from build123d import *

# Parameters (mm, degrees)
SKETCH4_W            = 31.4
SKETCH4_H            = 31.4
SKETCH4_W_2          = 25.4
SKETCH4_H_2          = 25.4
BOSS_EXTRUDE3_DEPTH  = 30
SKETCH5_W            = 31.4
SKETCH5_H            = 31.4
BOSS_EXTRUDE4_DEPTH  = 5
SKETCH6_W            = 31.4
SKETCH6_H            = 8
BOSS_EXTRUDE5_DEPTH  = 5
BOSS_EXTRUDE6_DEPTH  = 8
SKETCH8_R            = 9.5
BOSS_EXTRUDE7_DEPTH  = 8
SKETCH9_W            = 31.4
SKETCH9_H            = 10
BOSS_EXTRUDE8_DEPTH  = 5
SKETCH10_W           = 31.4
SKETCH10_H           = 10
BOSS_EXTRUDE9_DEPTH  = 13
SKETCH11_W           = 6.2
SKETCH11_H           = 10
BOSS_EXTRUDE10_DEPTH = 40
BOSS_EXTRUDE11_DEPTH = 3
SKETCH13_W           = 31.4
SKETCH13_H           = 31.4
CUT_EXTRUDE1_DEPTH   = 31.4
SKETCH15_W           = 31.4
SKETCH15_H           = 13
BOSS_EXTRUDE12_DEPTH = 12
SKETCH17_W           = 8
SKETCH17_H           = 31.4
BOSS_EXTRUDE13_DEPTH = 10
SKETCH18_R           = 3.5
BOSS_EXTRUDE14_DEPTH = 8
SKETCH19_W           = 3.6
SKETCH19_H           = 5
CUT_EXTRUDE2_DEPTH   = 31.4
CUT_EXTRUDE3_START   = 8
SKETCH8_2_R          = 9.5
CUT_EXTRUDE3_DEPTH   = 24
SKETCH20_W           = 8
SKETCH20_H           = 1
CUT_EXTRUDE4_DEPTH   = 26.4


with BuildPart() as part:
    # Sketch4 → Boss-Extrude3 (new body)
    with BuildSketch(Plane.XY):
        Rectangle(SKETCH4_W, SKETCH4_H)
        Rectangle(SKETCH4_W_2, SKETCH4_H_2, mode=Mode.SUBTRACT)
    extrude(amount=BOSS_EXTRUDE3_DEPTH)

    # Sketch5 → Boss-Extrude4 (add)
    with BuildSketch(Plane.XY.offset(30)):
        Rectangle(SKETCH5_W, SKETCH5_H)
    extrude(amount=BOSS_EXTRUDE4_DEPTH)

    # Sketch6 → Boss-Extrude5 (add)
    with BuildSketch(Plane.XY.offset(35)):
        Rectangle(SKETCH6_W, SKETCH6_H)
    extrude(amount=BOSS_EXTRUDE5_DEPTH)

    # Sketch7 → Boss-Extrude6 (add)
    with BuildSketch(Plane.XZ.offset(4)):
        with BuildLine():
            Line((-15.7, 40), (-15.7, 52))
            ThreePointArc((-15.7, 52), (-11.306601718, 62.606601718), (-0.7, 67))
            Line((-0.7, 67), (0.7, 67))
            ThreePointArc((0.7, 67), (11.306601718, 62.606601718), (15.7, 52))
            Line((15.7, 52), (15.7, 40))
            Line((15.7, 40), (-15.7, 40))
        make_face()
    extrude(amount=-BOSS_EXTRUDE6_DEPTH)

    # Sketch8 → Boss-Extrude7 (add)
    with BuildSketch(Plane.XZ.offset(4)):
        with Locations(Location((0, 52, 0), (0, 0, 180))):
            Circle(SKETCH8_R)
    boss_extrude7 = extrude(amount=BOSS_EXTRUDE7_DEPTH)

    # Mirror1: Boss-Extrude7 across plane
    add(boss_extrude7.mirror(Plane.ZX))

    # Sketch9 → Boss-Extrude8 (add)
    with BuildSketch(Plane(origin=(0, 15.7, 0), x_dir=(1, 0, 0), z_dir=(0, 1, 0))):
        with Locations((0, -27)):
            Rectangle(SKETCH9_W, SKETCH9_H)
    extrude(amount=BOSS_EXTRUDE8_DEPTH)

    # Sketch10 → Boss-Extrude9 (add)
    with BuildSketch(Plane(origin=(0, 15.7, 0), x_dir=(1, 0, 0), z_dir=(0, 1, 0))):
        with Locations((0, -17)):
            Rectangle(SKETCH10_W, SKETCH10_H)
    extrude(amount=BOSS_EXTRUDE9_DEPTH)

    # Sketch11 → Boss-Extrude10 (add)
    with BuildSketch(Plane(origin=(0, 20.7, 0), x_dir=(1, 0, 0), z_dir=(0, 1, 0))):
        with Locations((-12.6, -27)):
            Rectangle(SKETCH11_W, SKETCH11_H)
        with Locations((12.6, -27)):
            Rectangle(SKETCH11_W, SKETCH11_H)
    extrude(amount=BOSS_EXTRUDE10_DEPTH)

    # Sketch12 → Boss-Extrude11 (add)
    with BuildSketch(Plane.XY.offset(32)):
        Polygon((-15.7, 60.7), (-9.5, 60.7), (-9.5, 20.7), (9.5, 20.7), (9.5, 60.7), (15.7, 60.7), (15.7, 15.7), (-15.7, 15.7), align=None)
    extrude(amount=BOSS_EXTRUDE11_DEPTH)

    # Sketch13 → Cut-Extrude1 (cut)
    with BuildSketch(Plane.ZY.offset(15.7)):
        with Locations((15.7, 0)):
            Rectangle(SKETCH13_W, SKETCH13_H)
    extrude(amount=-CUT_EXTRUDE1_DEPTH, mode=Mode.SUBTRACT)

    # Sketch15 → Boss-Extrude12 (add)
    with BuildSketch(Plane(origin=(0, 0, 12), x_dir=(-1, 0, 0), z_dir=(0, 0, -1))):
        with Locations((0, 22.2)):
            Rectangle(SKETCH15_W, SKETCH15_H)
    extrude(amount=BOSS_EXTRUDE12_DEPTH)

    # Sketch17 → Boss-Extrude13 (add)
    with BuildSketch(Plane.XZ.offset(-15.7)):
        with Locations((-8, 15.7)):
            Rectangle(SKETCH17_W, SKETCH17_H)
    boss_extrude13 = extrude(amount=BOSS_EXTRUDE13_DEPTH)

    # Sketch18 → Boss-Extrude14 (add)
    with BuildSketch(Plane.ZY.offset(12)):
        with BuildLine():
            Line((31.4, 5.7), (0, 5.7))
            Line((0, 5.7), (0, -13.3))
            ThreePointArc((0, -13.3), (4.393398282, -23.906601718), (15, -28.3))
            Line((15, -28.3), (16.4, -28.3))
            ThreePointArc((16.4, -28.3), (27.006601718, -23.906601718), (31.4, -13.3))
            Line((31.4, -13.3), (31.4, 5.7))
        make_face()
        with Locations((15.7, -13.3)):
            Circle(SKETCH18_R, mode=Mode.SUBTRACT)
    boss_extrude14 = extrude(amount=-BOSS_EXTRUDE14_DEPTH)

    # Mirror3: Boss-Extrude13, Boss-Extrude14 across plane
    add(boss_extrude13.mirror(Plane(origin=(0, 0, 0), x_dir=(0, 0, 1), z_dir=(1, 0, 0))))
    add(boss_extrude14.mirror(Plane(origin=(0, 0, 0), x_dir=(0, 0, 1), z_dir=(1, 0, 0))))

    # Sketch19 → Cut-Extrude2 (cut)
    with BuildSketch(Plane(origin=(15.7, 0, 0), x_dir=(0, 0, -1), z_dir=(1, 0, 0))):
        with Locations((-33.2, -13.2)):
            Rectangle(SKETCH19_W, SKETCH19_H)
    extrude(amount=-CUT_EXTRUDE2_DEPTH, mode=Mode.SUBTRACT)

    # Sketch8_2 → Cut-Extrude3 (cut)
    with BuildSketch(Plane.XZ.offset(4).offset(CUT_EXTRUDE3_START)):
        with Locations(Location((0, 52, 0), (0, 0, 270))):
            Circle(SKETCH8_2_R)
    extrude(amount=-CUT_EXTRUDE3_DEPTH, mode=Mode.SUBTRACT)

    # Sketch20 → Cut-Extrude4 (cut)
    with BuildSketch(Plane.XZ.offset(10.7)):
        with Locations((0, 31.9)):
            Rectangle(SKETCH20_W, SKETCH20_H)
    extrude(amount=-CUT_EXTRUDE4_DEPTH, mode=Mode.SUBTRACT)


solid = part.part
Model file for the job. Use its own axes, mm. A direction names the side the tool comes from. Give positions to 0.01 mm unless a question says otherwise; leave off trailing zeros. Order: outer loops, then holes, each group sorted by start corner. A loop starts at its lowest first (then second) coordinate and runs counter-clockwise, first axis right, second up. Notation, with made-up numbers: M -36,-39 L 5,-39 A23 ccw 5,-14 Z; hole C 58.25,-37.75 d7. An arc over 180 degrees is marked long. Put each result on its own line as item: value. Start each with the question number.
(1) Pin check, flat tips, straight feed: pin 1 Ø3 at (x, z) = (-8, 46) entering from -Y; pin 2 Ø11 at (y, z) = (-13.3, 15.7) entering from +X; pin 3 Ø6 at (x, z) = (0.5, 17) entering from -Y. Stop position of each tip, or through.
(2) Tool access for faces 5 (the face through (-8, -12, 31.4)), 6 (the face through (0, 20.7, 28)), 7 (the face through (14, 2, 31.4)), 8 (the face through (-14, 15.7, 16)), 9 (the face through (-4, -6, 16)): list every direction of +Z, -Z, +X, -X, +Y, -Y with a clear straight run to the whole face (end or side of a thin tool).
(3) Band-saw the part on D-D on x = 2.5. Give the cut face in (y, z), then the cut area to 3 significant figures.
(4) Band-saw the part on A-A on y = 34. Give the cut face in (x, z).
(5) Band-saw the part on C-C on y = 1. Give the cut face in (x, z), then the cut area to 3 significant figures.
(6) Band-saw the part on B-B on x = -6. Give the cut face in (y, z), then the cut area to 3 significant figures.
(7) Pull direction X, two halves, no side cores. Call faces 1 (the face through (9.5, 40, 28)), 2 (the face through (12, -6, 15)), 3 (the face through (-15.7, 27, 28)), 4 (the face through (-8.06, -23.79, 4.28)): released by +X, released by -X, zero draft, split by the parting line, or undercut.
(8) Drill centre lines: L1, parallel to Y at x = 10.25, z = 15.7; L2, parallel to Z at x = 7, y = -13; L3, parallel to X at y = 0, z = 19.5. Where is each one in solid material? Low to high. Write a range as [from, to].
Results below:
1. pin 1: stops at y = -4
1. pin 2: stops at x = 12
1. pin 3: stops at y = 15.7
2. face 5: +Z, +X, -X, -Y
2. face 6: +Z, +Y
2. face 7: -Z, +X, -Y
2. face 8: -Z, -X, -Y
2. face 9: -Z, -Y
3. outline: M -10.7,32.4 L 15.7,32.4 L 15.7,0 L 28.7,0 L 28.7,22 L 20.7,22 L 20.7,35 L 4,35 L 4,42.83 L -4,42.83 L -4,35 L -10.7,35 Z; M -4,61.17 L 4,61.17 L 4,66.89 L -4,66.89 Z
3. area: 528 mm2
4. outline: M -15.7,22 L -9.5,22 L -9.5,35 L -15.7,35 Z; M 9.5,22 L 15.7,22 L 15.7,35 L 9.5,35 Z
5. outline: M -15.7,31.4 L -12,31.4 L -12,0 L -4,0 L -4,32.4 L 4,32.4 L 4,0 L 12,0 L 12,31.4 L 15.7,31.4 L 15.7,52 A15 ccw 0.7,67 L -0.7,67 A15 ccw -15.7,52 Z; hole C 0,52 d19
5. area: 1,230 mm2
6. outline: M -28.3,15 A15 ccw -13.3,0 L 28.7,0 L 28.7,22 L 20.7,22 L 20.7,35 L 4,35 L 4,44.63 L -4,44.63 L -4,35 L -10.7,35 L -10.7,31.4 L -13.3,31.4 A15 ccw -28.3,16.4 Z; M -4,59.37 L 4,59.37 L 4,66.03 L -4,66.03 Z; hole C -13.3,15.7 d7
6. area: 1,820 mm2
7. face 1: undercut
7. face 2: released by +X
7. face 3: released by -X
7. face 4: zero draft
8. L1: y = [-28.3, -16.8], [-9.8, 28.7]
8. L2: z = [0, 12.21], [19.19, 31.4]
8. L3: x = [-12, -4], [4, 12]
